The listing builds one solid part. Answer for the finished solid, in the listing's coordinates (mm). Face numbers are marked on the shaded views. A direction names the side the tool comes from. Round coordinates to 2 decimals unless told otherwise and drop trailing zeros. Write each loop counter-clockwise with the first axis right and the second up, starting at its lowest first coordinate (ties: lowest second). Pieces come first, ordered by that corner, then holes. Notation, with made-up numbers: (-4, 26.5) - (55, 26.5) arc R33 ccw to (55, 62.5) - close; hole circle Ø2 at (63, 28.25). An arc over 180 degrees is marked (long way). Use a Markdown table: item, result. Add a question column.
1) A cutting plane is placed at A-A (x = -54). Give the vertices of the cut face in (y, z), then the cut area to 3 significant figures.
2) Find the intervals of material crossed by probe 1 along Y at (x, z) = (-14, 3.75); probe 2 along Y at (x, z) = (13, 16.75); probe 3 along Z at (x, y) = (55.5, 9), in increasing order. Write a range as from..to.
3) Determine the mould class of the marked faces 4, 5 and 6 for opening direction Y: +Y half, -Y half, draft (parallel to the pull), parting line (faces both ways), or undercut.
4) A cutting plane is placed at B-B (y = 19.5). Give the vertices of the cut face in (x, z), then the cut area to 3 significant figures.
5) A cutting plane is placed at D-D (y = 12.25). Give the vertices of the cut face in (x, z).
6) A cutting plane is placed at C-C (z = 21.5). Give the vertices of the cut face in (x, y).
7) Each of these flat-tipped pins is pushed along its axis until it touches: P1, Ø3, axis at x = 17, y = 13.5, coming from the +Z side; P2, Ø2, axis at x = 4.5, y = 3.5, coming from the +Z side. Where does it stop, or does it pass through?
8) A tool of negligible diameter and unlimited length cuts with its end or side. For the marked faces 1, 2 and 3, from which of +Z, -Z, +X, -X, +Y, -Y can it reach the whole face along a straight path? Write none if from no direction.
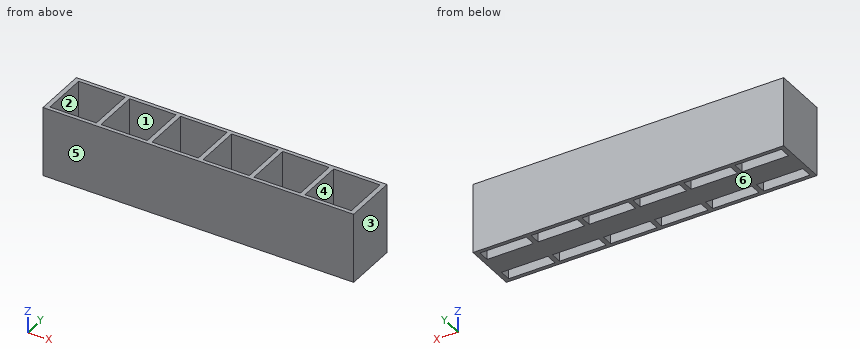
```python
from build123d import *

# Parameters (mm, degrees)
F0_W     = 134
F0_H     = 23.2
F0_W_2   = 20
F0_H_2   = 20
F1_DEPTH = 30
F2_W     = 132
F2_H     = 10
F3_DEPTH = 4


with BuildPart() as f1:
    # F0 (on Top) → F1 (new body)
    with BuildSketch(Plane.XY):
        with Locations((1, 11.6)):
            Rectangle(F0_W, F0_H)
        with Locations((-54, 11.6)):
            Rectangle(F0_W_2, F0_H_2, mode=Mode.SUBTRACT)
        with Locations((-32, 11.6)):
            Rectangle(F0_W_2, F0_H_2, mode=Mode.SUBTRACT)
        with Locations((-10, 11.6)):
            Rectangle(F0_W_2, F0_H_2, mode=Mode.SUBTRACT)
        with Locations((12, 11.6)):
            Rectangle(F0_W_2, F0_H_2, mode=Mode.SUBTRACT)
        with Locations((34, 11.6)):
            Rectangle(F0_W_2, F0_H_2, mode=Mode.SUBTRACT)
        with Locations((56, 11.6)):
            Rectangle(F0_W_2, F0_H_2, mode=Mode.SUBTRACT)
    extrude(amount=F1_DEPTH)

    # F2 (on Top) → F3 (join)
    with BuildSketch(Plane.XY):
        with Locations((1, 11.6)):
            Rectangle(F2_W, F2_H)
    extrude(amount=F3_DEPTH)


solid = f1.part
```
Entries:
| question | item | result |
|---|---|---|
| 1 | outline | (0, 0) - (1.6, 0) - (1.6, 30) - (0, 30) - close; (6.6, 0) - (16.6, 0) - (16.6, 4) - (6.6, 4) - close; (21.6, 0) - (23.2, 0) - (23.2, 30) - (21.6, 30) - close |
| 1 | area | 136 mm² |
| 2 | probe 1 | y = 0..1.6, 6.6..16.6, 21.6..23.2 |
| 2 | probe 2 | y = 0..1.6, 21.6..23.2 |
| 2 | probe 3 | z = 0..4 |
| 3 | face 4 | undercut |
| 3 | face 5 | -Y half |
| 3 | face 6 | draft |
| 4 | outline | (-66, 0) - (-64, 0) - (-64, 30) - (-66, 30) - close; (-44, 0) - (-42, 0) - (-42, 30) - (-44, 30) - close; (-22, 0) - (-20, 0) - (-20, 30) - (-22, 30) - close; (0, 0) - (2, 0) - (2, 30) - (0, 30) - close; (22, 0) - (24, 0) - (24, 30) - (22, 30) - close; (44, 0) - (46, 0) - (46, 30) - (44, 30) - close; (66, 0) - (68, 0) - (68, 30) - (66, 30) - close |
| 4 | area | 420 mm² |
| 5 | outline | (-66, 0) - (68, 0) - (68, 30) - (66, 30) - (66, 4) - (46, 4) - (46, 30) - (44, 30) - (44, 4) - (24, 4) - (24, 30) - (22, 30) - (22, 4) - (2, 4) - (2, 30) - (0, 30) - (0, 4) - (-20, 4) - (-20, 30) - (-22, 30) - (-22, 4) - (-42, 4) - (-42, 30) - (-44, 30) - (-44, 4) - (-64, 4) - (-64, 30) - (-66, 30) - close |
| 6 | outline | (-66, 0) - (68, 0) - (68, 23.2) - (-66, 23.2) - close; hole (-64, 1.6) - (-44, 1.6) - (-44, 21.6) - (-64, 21.6) - close; hole (-42, 1.6) - (-22, 1.6) - (-22, 21.6) - (-42, 21.6) - close; hole (-20, 1.6) - (0, 1.6) - (0, 21.6) - (-20, 21.6) - close; hole (2, 1.6) - (22, 1.6) - (22, 21.6) - (2, 21.6) - close; hole (24, 1.6) - (44, 1.6) - (44, 21.6) - (24, 21.6) - close; hole (46, 1.6) - (66, 1.6) - (66, 21.6) - (46, 21.6) - close |
| 7 | P1 | stops at z = 4 |
| 7 | P2 | passes through |
| 8 | face 1 | +Z, -Z |
| 8 | face 2 | +Z |
| 8 | face 3 | +Z, -Z, +X, +Y, -Y |
